Input: part model. Units: mm. Frame: model coordinates. A direction names the side the tool comes from. Coordinates: 2 decimals unless noted, no trailing zeros. Write each loop counter-clockwise with the first axis right and the second up, starting at its lowest first coordinate (ties: lowest second). Pieces come first, ordered by that corner, then holes. Notation, with made-up numbers: M -37.75,79 L 3.25,79 A11 ccw 3.25,100 Z; hole C 65,81 d2. An arc over 180 degrees is marked long. Use one line per item in the form item = value.
from build123d import *

# Parameters (mm, degrees)
SKETCH1_R             = 10
BOSS_EXTRUDE1_DEPTH   = 25
M5_TAPPED_HOLE1_D     = 4.2
M5_TAPPED_HOLE1_DEPTH = 13.7381927
M5_TAPPED_HOLE1_TIP   = 1.2618073
SKETCH18_R            = 10
SKETCH18_R_2          = 7.5
CUT_EXTRUDE1_DEPTH    = 5


with BuildPart() as part:
    # Sketch1 → Boss-Extrude1 (new body)
    with BuildSketch(Plane(origin=(0, 0, 0), x_dir=(1, 0, 0), z_dir=(0, 1, 0))):
        Circle(SKETCH1_R)
    extrude(amount=BOSS_EXTRUDE1_DEPTH)

    # M5 Tapped Hole1
    with Locations(Plane(origin=(0, 25, 0), x_dir=(1, 0, 0), z_dir=(0, 1, 0))):
        with Locations((0, 0)):
            Hole(M5_TAPPED_HOLE1_D / 2, depth=M5_TAPPED_HOLE1_DEPTH)
            with Locations((0, 0, -(M5_TAPPED_HOLE1_DEPTH + M5_TAPPED_HOLE1_TIP / 2))):  # 118° drill point
                Cone(0, M5_TAPPED_HOLE1_D / 2, M5_TAPPED_HOLE1_TIP, mode=Mode.SUBTRACT)

    # Sketch18 → Cut-Extrude1 (cut)
    with BuildSketch(Plane(origin=(0, 25, 0), x_dir=(1, 0, 0), z_dir=(0, 1, 0))):
        Circle(SKETCH18_R)
        Circle(SKETCH18_R_2, mode=Mode.SUBTRACT)
    extrude(amount=-CUT_EXTRUDE1_DEPTH, mode=Mode.SUBTRACT)


solid = part.part
(1) Pull-direction query (Z, two-part tool) for faces 1 (the flat face through (4, 20, -7)), 2 (the cylindrical face through (-2.003, 18.035, -0.631)), 3 (the cylindrical face through (-2.17, 9.86, 9.76)); classes: pulls with the +Z half, pulls with the -Z half, needs draft (parallel to the pull), parting line crosses it, or undercut.
Computed:
face_1 = needs draft
face_2 = undercut
face_3 = parting line crosses it
(2) Set-up query: faces 4 (the cylindrical face through (-7.493, 22.535, -0.33)), 5 (the flat face through (0, 0, 0)). Return all of +Z, -Z, +X, -X, +Y, -Y with unobstructed straight access to the full face (end or side cutting, diameter ignored); none if empty.
Computed:
face_4 = +Y
face_5 = +Z, -Z, +X, -X, -Y
(3) Section query B-B on y = 21. Return the cut outline in (x, z).
Computed:
outline = C 0,0 d15; hole C 0,0 d4.2
(4) First-contact query: pin 1 Ø1 at (y, z) = (8.5, -2.5) entering from +X; pin 2 Ø2.5 at (x, z) = (0, 0) entering from +Y. Flat tips, straight axial feed; report the tip coordinate or a pass-through.
Computed:
pin_1 = 9.8
pin_2 = 10.75
(5) Section query A-A on x = -2.5. Return the cut outline in (y, z), plus the area to 3 significant figures.
Computed:
outline = M 0,-9.68 L 20,-9.68 L 20,-7.07 L 25,-7.07 L 25,7.07 L 20,7.07 L 20,9.68 L 0,9.68 Z
area = 458 mm^2
(6) Section query D-D on y = 5.25. Return the cut outline in (x, z), plus the area to 3 significant figures.
Computed:
outline = C 0,0 d20
area = 314 mm^2
(7) Line query: probe 1 along Z at (x, y) = (0, 17); probe 2 along Y at (x, z) = (-1.5, 8); probe 3 along X at (y, z) = (17.5, -6.25). Output: solid intervals per line, ascending.
Computed:
probe_1 = -10 to -2.1, 2.1 to 10
probe_2 = 0 to 20
probe_3 = -7.81 to 7.81
(8) Section query C-C on z = 6.5. Return the cut outline in (x, y).
Computed:
outline = M -7.6,0 L 7.6,0 L 7.6,20 L 3.74,20 L 3.74,25 L -3.74,25 L -3.74,20 L -7.6,20 Z
